Source: CAD feature listing. Evaluate the final solid. Frame: model axes, mm. A direction names the side the tool comes from. Round coordinates to 2 decimals unless told otherwise and drop trailing zeros. Write each loop counter-clockwise with the first axis right and the second up, starting at its lowest first coordinate (ties: lowest second). Pieces come first, ordered by that corner, then holes. Notation, with made-up numbers: M 65,22.25 L 95,22.25 A22 ccw 95,47.25 Z; hole C 28,-22.75 d10. An arc over 180 degrees is marked long. Use a Markdown table: item, result.
```python
from build123d import *

# Parameters (mm, degrees)
SKETCH1_R                          = 57.15
SEAL_SEAT_HIEGHT_DEPTH             = 5.5372
SKETCH2_R                          = 57.15
SEAL_DIAPHRAM_HIEGHT_DEPTH         = 15.875
SEAL_START                         = 2
SKETCH3_R                          = 57.15
SEAL_SHOULDER_HIEGHT_DEPTH         = 2
SKETCH4_R                          = 57.15
BOTTOM_SEAL_CLEARANCE_DEPTH        = 2
SKETCH5_R                          = 11.1125
SEAL_SEAT_FIT_DEPTH                = 5.5372
SEAL_DIAPHRAM_CLEARANCE_DEPTH      = 2
SEAL_DIAPHRAM_CLEARANCE_DEPTH_BACK = 15.875
SKETCH6_R                          = 12.7
SKETCH7_R                          = 5.7625
SHAFT_CLEARANCE_DEPTH              = 2
M8_CLEARANCE_HOLE1_D               = 8.4


with BuildPart() as part:
    # Sketch1 → seal seat hieght (new body)
    with BuildSketch(Plane(origin=(0, 0, 0), x_dir=(1, 0, 0), z_dir=(0, 1, 0))):
        with Locations(Location((0, 0, 0), (0, 0, 270))):
            Circle(SKETCH1_R)
    extrude(amount=-SEAL_SEAT_HIEGHT_DEPTH)

    # Sketch2 → seal diaphram hieght (add)
    with BuildSketch(Plane.XZ.offset(5.5372)):
        with Locations(Location((0, 0, 0), (0, 0, 90))):
            Circle(SKETCH2_R)
    extrude(amount=SEAL_DIAPHRAM_HIEGHT_DEPTH)

    # Sketch3 → seal shoulder hieght (add)
    with BuildSketch(Plane(origin=(0, 0, 0), x_dir=(1, 0, 0), z_dir=(0, 1, 0)).offset(SEAL_START)):
        with Locations(Location((0, 0, 0), (0, 0, 270))):
            Circle(SKETCH3_R)
    extrude(amount=-SEAL_SHOULDER_HIEGHT_DEPTH)

    # Sketch4 → bottom seal clearance (add)
    with BuildSketch(Plane.XZ.offset(21.4122)):
        with Locations(Location((0, 0, 0), (0, 0, 90))):
            Circle(SKETCH4_R)
    extrude(amount=BOTTOM_SEAL_CLEARANCE_DEPTH)

    # Sketch5 → seal seat fit (cut)
    with BuildSketch(Plane(origin=(0, 0, 0), x_dir=(1, 0, 0), z_dir=(0, 1, 0))):
        with Locations(Location((0, 0, 0), (0, 0, 270))):
            Circle(SKETCH5_R)
    extrude(amount=-SEAL_SEAT_FIT_DEPTH, mode=Mode.SUBTRACT)

    # Sketch6 → seal diaphram clearance (cut, two sides: drawn at the far end of the back side and taken through both)
    with BuildSketch(Plane(origin=(0, -21.4122, 0), x_dir=(-1, 0, 0), z_dir=(0, -1, 0)).offset(-SEAL_DIAPHRAM_CLEARANCE_DEPTH_BACK)):
        with Locations(Location((0, 0, 0), (0, 0, 90))):
            Circle(SKETCH6_R)
    extrude(amount=SEAL_DIAPHRAM_CLEARANCE_DEPTH + SEAL_DIAPHRAM_CLEARANCE_DEPTH_BACK, mode=Mode.SUBTRACT)

    # Sketch7 → shaft clearance (cut)
    with BuildSketch(Plane(origin=(0, 0, 0), x_dir=(1, 0, 0), z_dir=(0, 1, 0))):
        with Locations(Location((0, 0, 0), (0, 0, 270))):
            Circle(SKETCH7_R)
    extrude(amount=SHAFT_CLEARANCE_DEPTH, mode=Mode.SUBTRACT)

    # M8 Clearance Hole1 (through all)
    with Locations(Plane(origin=(0, 2, 0), x_dir=(1, 0, 0), z_dir=(0, 1, 0))):
        with Locations((-44.45, 0), (0, 44.45), (44.45, 0), (0, -44.45)):
            Hole(M8_CLEARANCE_HOLE1_D / 2)


solid = part.part
```
Q1. First-contact query: pin 1 Ø6 at (y, z) = (-5, -23) entering from -X; pin 2 Ø1 at (y, z) = (-19.5, -43.5) entering from -X; pin 3 Ø11 at (x, z) = (0, -44.45) entering from -Y; pin 4 Ø18 at (x, z) = (-3, 0.5) entering from -Y. Flat tips, straight axial feed; report the tip coordinate or a pass-through.
Results are:
| item | result |
|---|---|
| pin 1 | x = -53.54 |
| pin 2 | x = -37.64 |
| pin 3 | y = -23.41 |
| pin 4 | y = -5.54 |
Q2. Section D-D on x = 46. Return loops of the section in (y, z).
Results are:
| item | result |
|---|---|
| outline | M -23.41,-33.91 L 2,-33.91 L 2,-3.9 L -23.41,-3.9 Z; M -23.41,3.9 L 2,3.9 L 2,33.91 L -23.41,33.91 Z |
Q3. Section A-A on z = 0. Return loops of the section in (x, y).
Results are:
| item | result |
|---|---|
| outline | M -57.15,-23.41 L -48.65,-23.41 L -48.65,2 L -57.15,2 Z; M -40.25,-23.41 L -12.7,-23.41 L -12.7,-5.54 L -11.11,-5.54 L -11.11,0 L -5.76,0 L -5.76,2 L -40.25,2 Z; M 5.76,0 L 11.11,0 L 11.11,-5.54 L 12.7,-5.54 L 12.7,-23.41 L 40.25,-23.41 L 40.25,2 L 5.76,2 Z; M 48.65,-23.41 L 57.15,-23.41 L 57.15,2 L 48.65,2 Z |
Q4. Section C-C on y = -21.5. Return loops of the section in (x, z).
Results are:
| item | result |
|---|---|
| outline | C 0,0 d114.3; hole C -44.45,0 d8.4; hole C 0,0 d25.4; hole C 0,-44.45 d8.4; hole C 0,44.45 d8.4; hole C 44.45,0 d8.4 |
Q5. Section B-B on x = 0. Return loops of the section in (y, z), plus the area to 3 significant figures.
Results are:
| item | result |
|---|---|
| outline | M -23.41,-57.15 L 2,-57.15 L 2,-48.65 L -23.41,-48.65 Z; M -23.41,-40.25 L 2,-40.25 L 2,-5.76 L 0,-5.76 L 0,-11.11 L -5.54,-11.11 L -5.54,-12.7 L -23.41,-12.7 Z; M -23.41,12.7 L -5.54,12.7 L -5.54,11.11 L 0,11.11 L 0,5.76 L 2,5.76 L 2,40.25 L -23.41,40.25 Z; M -23.41,48.65 L 2,48.65 L 2,57.15 L -23.41,57.15 Z |
| area | 1,880 mm^2 |
Q6. Reachability of faces 1 (the cylindrical face through (-7.7, -14.3, 10.1)), 2 (the flat face through (-1, -23.412, -14)) from +Z, -Z, +X, -X, +Y, -Y: full face, straight path, thin tool, end or side. Return the list, or none.
Results are:
| item | result |
|---|---|
| face 1 | -Y |
| face 2 | +Z, -Z, +X, -X, -Y |
Q7. Mould query, pull axis X, two halves, no side actions, for faces 3 (the cylindrical face through (-48.456, -10.884, -1.262)), 4 (the cylindrical face through (-2.513, -10.528, -57.095)), 5 (the flat face through (-12, 2, -1)). Classes: +X half, -X half, draft (parallel to the pull), parting line (faces both ways), or undercut.
Results are:
| item | result |
|---|---|
| face 3 | undercut |
| face 4 | parting line |
| face 5 | draft |
Q8. Line query: L1, parallel to X at y = -14.5, z = -4.5; L2, parallel to Z at x = 44.45, y = -17.25. Output: solid intervals per line, ascending.
Results are:
| item | result |
|---|---|
| L1 | -56.97 to -11.88, 11.88 to 56.97 |
| L2 | -35.92 to -4.2, 4.2 to 35.92 |
